The model under review builds one solid part; all positions refer to its coordinate system, in mm. A direction names the side the tool comes from. Give positions to 0.01 mm unless a question says otherwise; leave off trailing zeros. Order: outer loops, then holes, each group sorted by start corner. A loop starts at its lowest first (then second) coordinate and runs counter-clockwise, first axis right, second up. Notation, with made-up numbers: (84, 37.25) - (112, 37.25) arc R22 cw to (112, 44.25) - close; hole circle Ø7 at (-21, 56.25). An arc over 180 degrees is marked (long way). Use CSV: the item, a comma, the result in double quotes.
```python
from build123d import *

# Parameters (mm, degrees)
SKETCH_2_W      = 50
SKETCH_2_H      = 10
EXTRUDE_1_DEPTH = 15
SKETCH_3_W      = 3
SKETCH_3_H      = 42
EXTRUDE_2_DEPTH = 5
SKETCH_4_W      = 3
SKETCH_4_H      = 5
EXTRUDE_4_DEPTH = 5
EXTRUDE_5_DEPTH = 5


with BuildPart() as part:
    # 草图2 → 凸台-拉伸1 (new body)
    with BuildSketch(Plane.XY):
        Polygon((-29.132569558, 18.56468986), (-32.132569558, 18.56468986), (-32.132569558, -23.43531014), (-29.132569558, -23.43531014), (23.867430442, -23.43531014), (23.867430442, 18.56468986), align=None)
        with Locations((-4.132569558, 10.56468986)):
            Rectangle(SKETCH_2_W, SKETCH_2_H, mode=Mode.SUBTRACT)
        with Locations((-4.132569558, -2.43531014)):
            Rectangle(SKETCH_2_W, SKETCH_2_H, mode=Mode.SUBTRACT)
        with Locations((-4.132569558, -15.43531014)):
            Rectangle(SKETCH_2_W, SKETCH_2_H, mode=Mode.SUBTRACT)
    extrude(amount=EXTRUDE_1_DEPTH)

    # 草图3 → 凸台-拉伸2 (add)
    with BuildSketch(Plane(origin=(0, 0, 0), x_dir=(-1, 0, 0), z_dir=(0, 0, -1))):
        with Locations((30.632569558, -2.43531014)):
            Rectangle(SKETCH_3_W, SKETCH_3_H)
        with Locations((-22.367430442, -2.43531014)):
            Rectangle(SKETCH_3_W, SKETCH_3_H)
    extrude(amount=EXTRUDE_2_DEPTH)

    # 草图4 → 凸台-拉伸4 (add)
    with BuildSketch(Plane(origin=(0, 18.56468986, 0), x_dir=(1, 0, 0), z_dir=(0, 1, 0))):
        with Locations((-30.632569558, 2.5)):
            Rectangle(SKETCH_4_W, SKETCH_4_H)
        with Locations((22.367430442, 2.5)):
            Rectangle(SKETCH_4_W, SKETCH_4_H)
    extrude(amount=EXTRUDE_4_DEPTH)

    # 草图5 → 凸台-拉伸5 (add)
    with BuildSketch(Plane(origin=(0, 18.56468986, 0), x_dir=(1, 0, 0), z_dir=(0, 1, 0))):
        Polygon((23.867430442, 0), (20.867430442, 0), (-29.132569558, 0), (-32.132569558, 0), (-32.132569558, -15), (23.867430442, -15), align=None)
    extrude(amount=EXTRUDE_5_DEPTH)


solid = part.part
```
Item 1: Wall thickness on L1, parallel to Y at x = -4, z = 12.25; L2, parallel to X at y = -5.5, z = 0.25; L3, parallel to Z at x = -14, y = 17: over which ranges is each line inside the solid? List them lowest first.
Results list:
L1,"y = -23.44 to -20.44, -10.44 to -7.44, 2.56 to 5.56, 15.56 to 23.56"
L2,"x = -32.13 to -29.13, 20.87 to 23.87"
L3,"z = 0 to 15"
Item 2: Mouldability with a two-part tool opening along X and no side actions: class faces 4 (the face through (-4, 4, 0)), 5 (the face through (-31, 0, -5)), 6 (the face through (-32.133, 0, 5)) as pulls with the +X half, pulls with the -X half, needs draft (parallel to the pull), parting line crosses it, or undercut.
Results list:
face 4,"undercut"
face 5,"needs draft"
face 6,"pulls with the -X half"
Item 3: Take a section at D-D, the plane z = -1.75. Give the boundary of the cut face in (x, y).
Results list:
outline,"(-32.13, -23.44) - (-29.13, -23.44) - (-29.13, 23.56) - (-32.13, 23.56) - close; (20.87, -23.44) - (23.87, -23.44) - (23.87, 23.56) - (20.87, 23.56) - close"
Item 4: Tool access review of faces 1 (the face through (-5, 23.565, 7)), 2 (the face through (-4, 2.565, 7)), 3 (the face through (-4, -9, 0)): name each direction out of +Z, -Z, +X, -X, +Y, -Y from which nothing blocks a thin tool from reaching the whole face with its end or side.
Results list:
face 1,"+Z, -Z, +X, -X, +Y"
face 2,"+Z, -Z"
face 3,"-Z, +Y, -Y"
Item 5: Clearance check with a flat-ended pin moving along its axis: pin 1 (8 mm diameter, centred on x = -15.5, y = 0, fed in from -Z). State where the tip first meets the part, or that it passes through.
Results list:
pin 1,"stops at z = 0"
Item 6: Take a section at C-C, the plane y = 8.5. Give the boundary of the cut face in (x, z), and give its area (3 significant figures).
Results list:
outline,"(-32.13, -5) - (-29.13, -5) - (-29.13, 15) - (-32.13, 15) - close; (20.87, -5) - (23.87, -5) - (23.87, 15) - (20.87, 15) - close"
area,"120 mm2"
Item 7: Take a section at B-B, the plane z = 2. Give the boundary of the cut face in (x, y).
Results list:
outline,"(-32.13, -23.44) - (23.87, -23.44) - (23.87, 23.56) - (-32.13, 23.56) - close; hole (-29.13, -20.44) - (20.87, -20.44) - (20.87, -10.44) - (-29.13, -10.44) - close; hole (-29.13, -7.44) - (20.87, -7.44) - (20.87, 2.56) - (-29.13, 2.56) - close; hole (-29.13, 5.56) - (20.87, 5.56) - (20.87, 15.56) - (-29.13, 15.56) - close"
Item 8: Take a section at A-A, the plane x = -17. Give the boundary of the cut face in (y, z).
Results list:
outline,"(-23.44, 0) - (-20.44, 0) - (-20.44, 15) - (-23.44, 15) - close; (-10.44, 0) - (-7.44, 0) - (-7.44, 15) - (-10.44, 15) - close; (2.56, 0) - (5.56, 0) - (5.56, 15) - (2.56, 15) - close; (15.56, 0) - (23.56, 0) - (23.56, 15) - (15.56, 15) - close"
